```python
from build123d import *

# Parameters (mm, degrees)
CUT_SWEEP1_START   = -10.440114653
CUT_SWEEP1_DEPTH   = 20.880229306
CIRPATTERN1_COUNT  = 8
SKETCH5_R          = 7.9375
CUT_EXTRUDE1_DEPTH = 68.58
FILLET1_R          = 1.5875
FILLET2_R          = 3.175
FILLET3_R          = 25.4
FILLET4_R          = 6.35


# Read off the part's stored shape, not the designer's step: Cut-Sweep1
with BuildPart() as part:
    # Sweep2: sweep along a path in Sketch3
    with BuildLine(Plane(origin=(0, 0, 0), x_dir=(0, 0, -1), z_dir=(1, 0, 0))) as sweep2_path:
        Line((0, 0), (117.475, 0))
    # Sketch1 → Sweep2 (sweep)
    with BuildSketch(Plane.XY):
        Polygon((15.24, -6.312614691), (15.24, 6.312614691), (6.312614691, 15.24), (-6.312614691, 15.24), (-15.24, 6.312614691), (-15.24, -6.312614691), (-6.312614691, -15.24), (6.312614691, -15.24), align=None)
    sweep(path=sweep2_path.line)

    # Cut-Sweep1 outline → Cut-Sweep1 (cut)
    with BuildSketch(Plane.YZ.offset(CUT_SWEEP1_START)):
        with BuildLine():
            Line((15.24, -111.125), (15.24, -63.5))
            add(Edge.make_bspline(
                [(15.24, -63.5), (12.515117075, -71.124082686), (11.1125, -79.21695815), (11.1125, -95.40804185), (12.515117075, -103.500917314), (15.24, -111.125)],
                knots=[0, 0, 0, 0, 0.5, 0.5, 1, 1, 1, 1], degree=3))
        make_face()
    cut_sweep1 = extrude(amount=CUT_SWEEP1_DEPTH, mode=Mode.SUBTRACT)

    # CirPattern1: Cut-Sweep1 ×8 about axis
    cirpattern1_axis = Axis((0, 0, 0), (0, 0, -1))
    for i in range(1, CIRPATTERN1_COUNT):
        add(cut_sweep1.rotate(cirpattern1_axis, i * 360 / CIRPATTERN1_COUNT), mode=Mode.SUBTRACT)

    # Sketch5 → Cut-Extrude1 (cut)
    with BuildSketch(Plane(origin=(0, 0, -117.475), x_dir=(-1, 0, 0), z_dir=(0, 0, -1))):
        Circle(SKETCH5_R)
    extrude(amount=-CUT_EXTRUDE1_DEPTH, mode=Mode.SUBTRACT)

    # Fillet1
    fillet1_edges = [part.edges().sort_by_distance(p)[0] for p in [
        (10.776307345, -10.776307345, -117.475),
        (15.24, 0, -117.475),
        (10.776307345, 10.776307345, -117.475),
        (0, 15.24, -117.475),
        (-10.776307345, 10.776307345, -117.475),
        (-15.24, 0, -117.475),
        (-10.776307345, -10.776307345, -117.475),
        (0, -15.24, -117.475),
    ]]
    fillet(fillet1_edges, radius=FILLET1_R)

    # Fillet2
    fillet2_edges = [part.edges().sort_by_distance(p)[0] for p in [
        (15.24, 0, 0),
        (10.776307345, 10.776307345, 0),
        (0, 15.24, 0),
        (-10.776307345, 10.776307345, 0),
        (-15.24, 0, 0),
        (-10.776307345, -10.776307345, 0),
        (0, -15.24, 0),
        (10.776307345, -10.776307345, 0),
    ]]
    fillet(fillet2_edges, radius=FILLET2_R)

    # Fillet3
    fillet3_edges = [part.edges().sort_by_distance(p)[0] for p in [
        (10.776307345, 10.776307345, -63.5),
        (15.24, 0, -63.5),
        (10.776307345, -10.776307345, -63.5),
        (0, -15.24, -63.5),
        (-10.776307345, -10.776307345, -63.5),
        (-15.24, 0, -63.5),
        (-10.776307345, 10.776307345, -63.5),
        (0, 15.24, -63.5),
    ]]
    fillet(fillet3_edges, radius=FILLET3_R)

    # Fillet4
    fillet4_edges = [part.edges().sort_by_distance(p)[0] for p in [
        (-10.776307345, -10.776307345, -111.125),
        (0, -15.24, -111.125),
        (10.776307345, -10.776307345, -111.125),
        (15.24, 0, -111.125),
        (10.776307345, 10.776307345, -111.125),
        (0, 15.24, -111.125),
        (-10.776307345, 10.776307345, -111.125),
        (-15.24, 0, -111.125),
    ]]
    fillet(fillet4_edges, radius=FILLET4_R)


solid = part.part
```
Check sheet for the modelled part. Datum: model origin and axes. Units: mm. Give positions to 0.01 mm unless a question says otherwise; leave off trailing zeros. Write each loop counter-clockwise with the first axis right and the second up, starting at its lowest first coordinate (ties: lowest second). Pieces come first, ordered by that corner, then holes. Notation, with made-up numbers: (81, 86.25) - (136, 86.25) arc R18 cw to (136, 95.25) - close; hole circle Ø3 at (23, 75.25). An arc over 180 degrees is marked (long way). Answer as a JSON object with one key per item and string values. Group by question number.
1) Thickness scan on probe 1 along Y at (x, z) = (-9.5, -14.5); probe 2 along X at (y, z) = (4, -87); probe 3 along X at (y, z) = (-2.5, -77). Record the ranges inside material, lowest first. Write a range as from..to.
2) Release check for a two-part mould opening along Y. For faces 1 (the face through (10.84, 10.71, -114.07)), 2 (the face through (6, 6, -117.475)), 3 (the face through (1.72, -7.75, -83.67)) record: pulls with the +Y half, pulls with the -Y half, needs draft (parallel to the pull), parting line crosses it, or undercut.
3) Sectioned sample at A-A (z = -43.5). Record the cut outline in (x, y).
4) Depth check by flat-ended pin: P1, Ø10, axis at x = -0.5, y = -2.5, coming from the -Z side (3 decimals); P2, Ø4, axis at y = -8, z = -88, coming from the +X side; P3, Ø1, axis at x = -8, z = -88, coming from the -Y side. Enter the tip coordinate at first touch or a pass-through.
Geometry results:
{
 "1": {"probe 1": "y = -12.05..12.05", "probe 2": "x = -11.11..-6.86, 6.86..11.11", "probe 3": "x = -11.87..-7.53, 7.53..11.87"},
 "2": {"face 1": "pulls with the +Y half", "face 2": "needs draft", "face 3": "undercut"},
 "3": {"outline": "(-15.24, -6.31) - (-6.31, -15.24) - (6.31, -15.24) - (15.24, -6.31) - (15.24, 6.31) - (6.31, 15.24) - (-6.31, 15.24) - (-15.24, 6.31) - close"},
 "4": {"P1": "stops at z = -48.895", "P2": "stops at x = 9.72", "P3": "stops at y = -8.22"}
}
